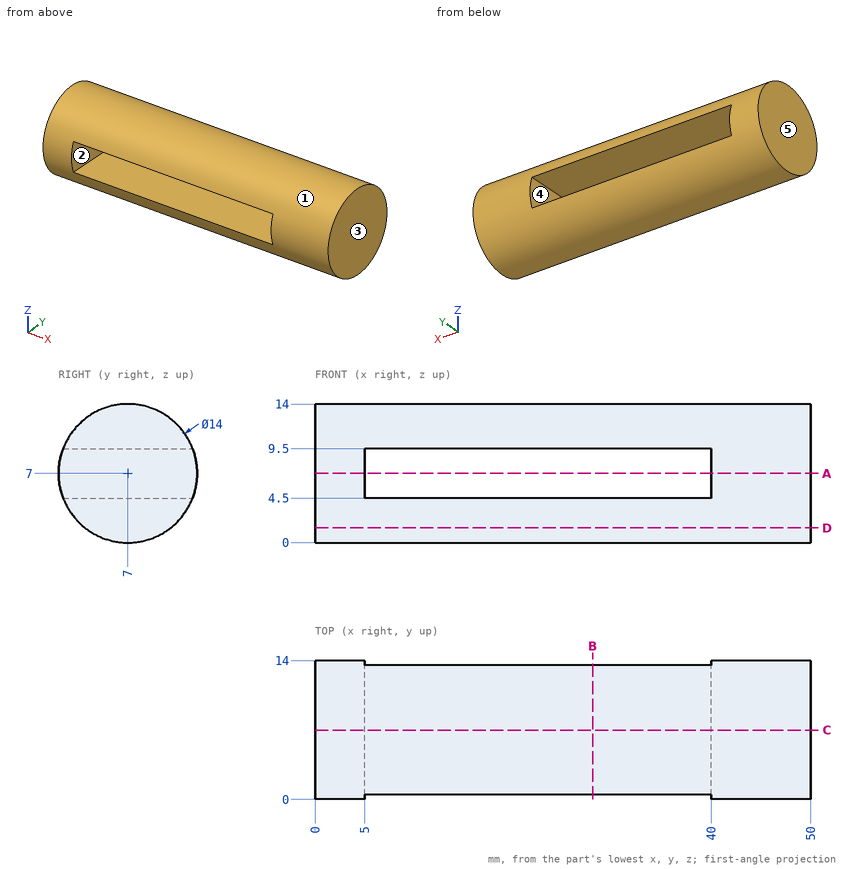
Can you work these out from the drawing? Everything is in mm from the part's minimum corner. A direction names the side the tool comes from. Coordinates: 2 decimals unless noted, no trailing zeros. Loops run counter-clockwise (first coordinate to the right, second up) from the corner with the lowest first, then second, coordinate; pieces in that order, holes last.
1. Imagine slicing it at B-B, the plane x = 28. Please give me the cut outline in (y, z), and give its area (3 significant figures).
2. I need wall thicknesses on L1, parallel to X at y = 2.75, z = 6.25; L2, parallel to Z at x = 8.5, y = 4; L3, parallel to Z at x = 30.5, y = 4.75. Which ranges of each line are inside material? Lowest first, please.
3. For the marked faces 1 and 2, which set-ups out of +Z, -Z, +X, -X, +Y, -Y let a thin tool reach every point of the face, with its end or its side?
4. Imagine slicing it at D-D, the plane z = 1.5. Please give me the cut outline in (x, y).
5. If we mould it in two halves opening along X, with no side actions, what happens to the marked faces 3, 4 and 5? For each: pulls with the +X half, pulls with the -X half, needs draft (parallel to the pull), parting line crosses it, or undercut.
6. Imagine slicing it at C-C, the plane y = 7. Please give me the cut outline in (x, z).
7. For P1, Ø1.5, axis at x = 26.5, y = 12.5, coming from the -Z side; P2, Ø1.5, axis at x = 44.5, y = 3.5, coming from the +Z side; P3, Ø4, axis at x = 27, y = 4.5, coming from the -Z side, each with a flat end and sliding along its axis, tell me the tip position at first contact or that it passes through.
8. Imagine slicing it at A-A, the plane z = 7. Please give me the cut outline in (x, y), and give its area (3 significant figures).
Taken from the geometry:
1. outline: (0.46, 4.5) arc R7 ccw to (13.54, 4.5) - close; (0.46, 9.5) - (13.54, 9.5) arc R7 ccw to start
1. area: 85.5 mm2
2. L1: x = 0 to 5, 40 to 50
2. L2: z = 0.68 to 4.5, 9.5 to 13.32
2. L3: z = 0.37 to 4.5, 9.5 to 13.63
3. face 1: +X, -X
3. face 2: +Y, -Y
4. outline: (0, 2.67) - (50, 2.67) - (50, 11.33) - (0, 11.33) - close
5. face 3: pulls with the +X half
5. face 4: undercut
5. face 5: pulls with the -X half
6. outline: (0, 0) - (50, 0) - (50, 14) - (0, 14) - close; hole (5, 4.5) - (40, 4.5) - (40, 9.5) - (5, 9.5) - close
7. P1: stops at z = 1.86
7. P2: stops at z = 13.44
7. P3: stops at z = 0.02
8. outline: (0, 0) - (5, 0) - (5, 14) - (0, 14) - close; (40, 0) - (50, 0) - (50, 14) - (40, 14) - close
8. area: 210 mm2
